Part model, mm, in its own coordinate system. A direction names the side the tool comes from. Coordinates: 2 decimals unless noted, no trailing zeros. Order: outer loops, then holes, each group sorted by start corner. A loop starts at its lowest first (then second) coordinate and runs counter-clockwise, first axis right, second up.
from build123d import *

# Parameters (mm, degrees)
SKETCH_8_R           = 16
EXTRUDE_1_DEPTH      = 48.3
SKETCH_9_R           = 9.5
EXTRUDE_2_DEPTH      = 1.7
SKETCH_10_R          = 5
EXTRUDE_3_DEPTH      = 19.3
CUT_EXTRUDE_8_DEPTH  = 3
SKETCH_13_R          = 1.5
CUT_EXTRUDE_9_DEPTH  = 6
SKETCH_14_R          = 8
CUT_EXTRUDE_10_DEPTH = 1.2
SKETCH_15_R          = 2.5
CUT_EXTRUDE_11_DEPTH = 20
SKETCH_16_R          = 1.5
CUT_EXTRUDE_12_DEPTH = 4
SKETCH_17_W          = 1.387391921
SKETCH_17_H          = 0.126778365
CHAMFER_1_SIZE       = 0.5


with BuildPart() as part:
    # 草图8 → 凸台-拉伸1 (new body)
    with BuildSketch(Plane.XY):
        with Locations(Location((0, 0, 0), (0, 0, 180))):
            Circle(SKETCH_8_R)
    extrude(amount=EXTRUDE_1_DEPTH)

    # 草图9 → 凸台-拉伸2 (add)
    with BuildSketch(Plane.XY.offset(48.3)):
        Circle(SKETCH_9_R)
    extrude(amount=EXTRUDE_2_DEPTH)

    # 草图10 → 凸台-拉伸3 (add)
    with BuildSketch(Plane.XY.offset(50)):
        Circle(SKETCH_10_R)
    extrude(amount=EXTRUDE_3_DEPTH)

    # 切除-拉伸7 cone 1 section (through the dimple's axis) → 切除-拉伸7 (revolve, cut)
    with BuildSketch(Plane(origin=(0, 0, 69.3), x_dir=(0, -1, 0), z_dir=(1, 0, 0))):
        Polygon((0, 0), (0.813334859, 0), (0, 1.301607858), align=None)
    revolve(axis=Axis((0, 0, 69.3), (0, 0, -1)), mode=Mode.SUBTRACT)

    # 草图12 → 切除-拉伸8 (cut)
    with BuildSketch(Plane(origin=(0, 3.2, 0), x_dir=(1, 0, 0), z_dir=(0, 1, 0))):
        with BuildLine():
            Line((-1.5, -64.8), (-1.5, -55.8))
            ThreePointArc((-1.5, -55.8), (0, -54.3), (1.5, -55.8))
            Line((1.5, -55.8), (1.5, -64.8))
            ThreePointArc((1.5, -64.8), (0, -66.3), (-1.5, -64.8))
        make_face()
    extrude(amount=CUT_EXTRUDE_8_DEPTH, mode=Mode.SUBTRACT)

    # 草图13 → 切除-拉伸9 (cut)
    with BuildSketch(Plane.XY.offset(48.3)):
        with Locations((0, 13)):
            Circle(SKETCH_13_R)
        with Locations((-13, 0)):
            Circle(SKETCH_13_R)
        with Locations((0, -13)):
            Circle(SKETCH_13_R)
        with Locations((13, 0)):
            Circle(SKETCH_13_R)
    extrude(amount=-CUT_EXTRUDE_9_DEPTH, mode=Mode.SUBTRACT)

    # 草图14 → 切除-拉伸10 (cut)
    with BuildSketch(Plane(origin=(0, 0, 0), x_dir=(-1, 0, 0), z_dir=(0, 0, -1))):
        Circle(SKETCH_14_R)
    extrude(amount=-CUT_EXTRUDE_10_DEPTH, mode=Mode.SUBTRACT)

    # 草图15 → 切除-拉伸11 (cut)
    with BuildSketch(Plane(origin=(0, 0, 0), x_dir=(-1, 0, 0), z_dir=(0, 0, -1))):
        Circle(SKETCH_15_R)
    extrude(amount=-CUT_EXTRUDE_11_DEPTH, mode=Mode.SUBTRACT)

    # 草图16 → 切除-拉伸12 (cut)
    with BuildSketch(Plane(origin=(0, 0, 0), x_dir=(-1, 0, 0), z_dir=(0, 0, -1))):
        with Locations((0, 11)):
            Circle(SKETCH_16_R)
        with Locations((11, 0)):
            Circle(SKETCH_16_R)
        with Locations((0, -11)):
            Circle(SKETCH_16_R)
        with Locations((-11, 0)):
            Circle(SKETCH_16_R)
    extrude(amount=-CUT_EXTRUDE_12_DEPTH, mode=Mode.SUBTRACT)

    # 草图17 → 切除-旋转1 (revolve, cut)
    with BuildSketch(Plane(origin=(0, 0, 0), x_dir=(1, 0, 0), z_dir=(0, 1, 0)), mode=Mode.PRIVATE) as cut_revolve_1_sk:
        with Locations((16.513931417, -37.236610818)):
            Rectangle(SKETCH_17_W, SKETCH_17_H)
    revolve(cut_revolve_1_sk.sketch.rotate(Axis((0, 0, 69.3), (0, 0, -1)), 180), axis=Axis((0, 0, 69.3), (0, 0, -1)), mode=Mode.SUBTRACT)

    # 倒角1
    chamfer_1_edges = [part.edges().sort_by_distance(p)[0] for p in [
        (-5, 0, 69.3),
    ]]
    chamfer(chamfer_1_edges, length=CHAMFER_1_SIZE)


solid = part.part
Q1. Pin check, flat tips, straight feed: pin 1 Ø0.9 at (x, z) = (0.5, 60.5) entering from +Y; pin 2 Ø6 at (y, z) = (11, 33) entering from +X; pin 3 Ø5 at (x, y) = (0, -13) entering from +Z. Stop position of each tip, or through.
Results list:
pin 1: stops at y = 3.2
pin 2: stops at x = 13.86
pin 3: stops at z = 48.3
Q2. Mould opens along X. For faces 1 (the face through (3.47, 15.62, 42.72)), 2 (the face through (-0.325, 11.536, 45.342)), 3 (the face through (0, -1, 69.3)) say: pulls with the +X half, pulls with the -X half, needs draft (parallel to the pull), parting line crosses it, or undercut.
Results list:
face 1: parting line crosses it
face 2: undercut
face 3: needs draft
Q3. Which spindle directions (+Z, -Z, +X, -X, +Y, -Y) get a long thin tool onto all of the face, cutting with end or side? Do faces 4 (the face through (0, 4.1, 66.3)), 5 (the face through (13, 0, 42.3)), 6 (the face through (0.54, -2.44, 10.47)). Say none if no direction does.
Results list:
face 4: +Y
face 5: +Z
face 6: -Z
Q4. Cut at C-C on z = 21. Write the cut outline in (x, y).
Results list:
outline: circle Ø32 at (0, 0)
Q5. Cut at B-B on x = -6.5. Write the cut outline in (y, z).
Results list:
outline: (-14.62, 0) - (-4.66, 0) - (-4.66, 1.2) - (4.66, 1.2) - (4.66, 0) - (14.62, 0) - (14.62, 37.17) - (14.42, 37.17) - (14.42, 37.3) - (14.62, 37.3) - (14.62, 48.3) - (6.93, 48.3) - (6.93, 50) - (-6.93, 50) - (-6.93, 48.3) - (-14.62, 48.3) - (-14.62, 37.3) - (-14.42, 37.3) - (-14.42, 37.17) - (-14.62, 37.17) - close
Q6. Wall check: line 1 along Y through (x, z) = (0, 45.05); line 2 along Y through (x, z) = (0, 1.85); line 3 along Z through (x, y) = (-11.5, 4). Give the ranges that are in metal, low to high.
Results list:
line 1: y = -16 to -14.5, -11.5 to 11.5, 14.5 to 16
line 2: y = -16 to -12.5, -9.5 to -2.5, 2.5 to 9.5, 12.5 to 16
line 3: z = 0 to 48.3
Q7. Cut at A-A on z = 46.5. Write the cut outline in (x, y), and give its area (3 significant figures).
Results list:
outline: circle Ø32 at (0, 0); hole circle Ø3 at (-13, 0); hole circle Ø3 at (0, -13); hole circle Ø3 at (0, 13); hole circle Ø3 at (13, 0)
area: 776 mm2
